```python
from build123d import *

# Parameters (mm, degrees)
SKETCH1_R           = 2
BOSS_EXTRUDE1_DEPTH = 200


with BuildPart() as part:
    # Sketch1 → Boss-Extrude1 (new body)
    with BuildSketch(Plane(origin=(0, 0, 0), x_dir=(1, 0, 0), z_dir=(0, 1, 0))):
        with BuildLine():
            Line((2.824264069, 15.973654403), (5.128427125, 13.669491347))
            ThreePointArc((5.128427125, 13.669491347), (5.99551813, 12.371797952), (6.3, 10.841064222))
            Line((6.3, 10.841064222), (6.3, 9.158935778))
            ThreePointArc((6.3, 9.158935778), (5.99551813, 7.628202048), (5.128427125, 6.330508653))
            Line((5.128427125, 6.330508653), (2.824264069, 4.026345597))
            ThreePointArc((2.824264069, 4.026345597), (2.170389941, 3.896281946), (1.8, 4.450609665))
            Line((1.8, 4.450609665), (1.8, 7))
            ThreePointArc((1.8, 7), (1.653553391, 7.353553391), (1.3, 7.5))
            Line((1.3, 7.5), (0.5, 7.5))
            ThreePointArc((0.5, 7.5), (0.146446609, 7.353553391), (0, 7))
            Line((0, 7), (0, 2))
            ThreePointArc((0, 2), (0.585786438, 0.585786438), (2, 0))
            Line((2, 0), (7, 0))
            ThreePointArc((7, 0), (7.353553391, 0.146446609), (7.5, 0.5))
            Line((7.5, 0.5), (7.5, 1.3))
            ThreePointArc((7.5, 1.3), (7.353553391, 1.653553391), (7, 1.8))
            Line((7, 1.8), (4.450609665, 1.8))
            ThreePointArc((4.450609665, 1.8), (3.896281946, 2.170389941), (4.026345597, 2.824264069))
            Line((4.026345597, 2.824264069), (6.330508653, 5.128427125))
            ThreePointArc((6.330508653, 5.128427125), (7.628202048, 5.99551813), (9.158935778, 6.3))
            Line((9.158935778, 6.3), (10.841064222, 6.3))
            ThreePointArc((10.841064222, 6.3), (12.371797952, 5.99551813), (13.669491347, 5.128427125))
            Line((13.669491347, 5.128427125), (15.973654403, 2.824264069))
            ThreePointArc((15.973654403, 2.824264069), (16.103718054, 2.170389941), (15.549390335, 1.8))
            Line((15.549390335, 1.8), (13, 1.8))
            ThreePointArc((13, 1.8), (12.646446609, 1.653553391), (12.5, 1.3))
            Line((12.5, 1.3), (12.5, 0.5))
            ThreePointArc((12.5, 0.5), (12.646446609, 0.146446609), (13, 0))
            Line((13, 0), (18, 0))
            ThreePointArc((18, 0), (19.414213562, 0.585786438), (20, 2))
            Line((20, 2), (20, 7))
            ThreePointArc((20, 7), (19.853553391, 7.353553391), (19.5, 7.5))
            Line((19.5, 7.5), (18.7, 7.5))
            ThreePointArc((18.7, 7.5), (18.346446609, 7.353553391), (18.2, 7))
            Line((18.2, 7), (18.2, 4.450609665))
            ThreePointArc((18.2, 4.450609665), (17.829610059, 3.896281946), (17.175735931, 4.026345597))
            Line((17.175735931, 4.026345597), (14.871572875, 6.330508653))
            ThreePointArc((14.871572875, 6.330508653), (14.00448187, 7.628202048), (13.7, 9.158935778))
            Line((13.7, 9.158935778), (13.7, 10.841064222))
            ThreePointArc((13.7, 10.841064222), (14.00448187, 12.371797952), (14.871572875, 13.669491347))
            Line((14.871572875, 13.669491347), (17.175735931, 15.973654403))
            ThreePointArc((17.175735931, 15.973654403), (17.829610059, 16.103718054), (18.2, 15.549390335))
            Line((18.2, 15.549390335), (18.2, 13))
            ThreePointArc((18.2, 13), (18.346446609, 12.646446609), (18.7, 12.5))
            Line((18.7, 12.5), (19.5, 12.5))
            ThreePointArc((19.5, 12.5), (19.853553391, 12.646446609), (20, 13))
            Line((20, 13), (20, 18))
            ThreePointArc((20, 18), (19.414213562, 19.414213562), (18, 20))
            Line((18, 20), (13, 20))
            ThreePointArc((13, 20), (12.646446609, 19.853553391), (12.5, 19.5))
            Line((12.5, 19.5), (12.5, 18.7))
            ThreePointArc((12.5, 18.7), (12.646446609, 18.346446609), (13, 18.2))
            Line((13, 18.2), (15.549390335, 18.2))
            ThreePointArc((15.549390335, 18.2), (16.103718054, 17.829610059), (15.973654403, 17.175735931))
            Line((15.973654403, 17.175735931), (13.669491347, 14.871572875))
            ThreePointArc((13.669491347, 14.871572875), (12.371797952, 14.00448187), (10.841064222, 13.7))
            Line((10.841064222, 13.7), (9.158935778, 13.7))
            ThreePointArc((9.158935778, 13.7), (7.628202048, 14.00448187), (6.330508653, 14.871572875))
            Line((6.330508653, 14.871572875), (4.026345597, 17.175735931))
            ThreePointArc((4.026345597, 17.175735931), (3.896281946, 17.829610059), (4.450609665, 18.2))
            Line((4.450609665, 18.2), (7, 18.2))
            ThreePointArc((7, 18.2), (7.353553391, 18.346446609), (7.5, 18.7))
            Line((7.5, 18.7), (7.5, 19.5))
            ThreePointArc((7.5, 19.5), (7.353553391, 19.853553391), (7, 20))
            Line((7, 20), (2, 20))
            ThreePointArc((2, 20), (0.585786438, 19.414213562), (0, 18))
            Line((0, 18), (0, 13))
            ThreePointArc((0, 13), (0.146446609, 12.646446609), (0.5, 12.5))
            Line((0.5, 12.5), (1.3, 12.5))
            ThreePointArc((1.3, 12.5), (1.653553391, 12.646446609), (1.8, 13))
            Line((1.8, 13), (1.8, 15.549390335))
            ThreePointArc((1.8, 15.549390335), (2.170389941, 16.103718054), (2.824264069, 15.973654403))
        make_face()
        with Locations(Location((10, 10, 0), (0, 0, 270))):
            Circle(SKETCH1_R, mode=Mode.SUBTRACT)
    extrude(amount=-BOSS_EXTRUDE1_DEPTH)


solid = part.part
```
Model file for the job. Use its own axes, mm. Round coordinates to 2 decimals unless told otherwise and drop trailing zeros. One line per item, written item: value.
(1) Two-plate mould, pull along X, no slides. Class faces 1 (the flat face through (20, -99, -4)), 2 (the cylindrical face through (12, -99, -10)), 3 (the flat face through (4, -99, 0)), 4 (the flat face through (0, -99, -5)): pulls with the +X half, pulls with the -X half, needs draft (parallel to the pull), parting line crosses it, or undercut.
Values follow:
face 1: pulls with the +X half
face 2: undercut
face 3: needs draft
face 4: pulls with the -X half
(2) Drop flat-ended pins along their axis: P1, Ø1.9, axis at y = -143, z = -10.5, coming from the +X side; P2, Ø0.9, axis at x = 1, y = -79.5, coming from the -Z side; P3, Ø0.8, axis at x = 10, y = -124.5, coming from the -Z side; P4, Ø3, axis at x = 10, z = -10, coming from the -Y side. Give the stop position or say it passes through.
Values follow:
P1: stops at x = 13.75
P2: stops at z = -19.92
P3: stops at z = -13.7
P4: passes through
(3) Wall check: probe 1 along Z at (x, y) = (15.5, -31); probe 2 along Z at (x, y) = (12.75, -182.5); probe 3 along X at (y, z) = (-61.5, -10). Give the ranges that are in metal, low to high.
Values follow:
probe 1: z = -20 to -18.2, -16.7 to -14.3, -5.7 to -3.3, -1.8 to 0
probe 2: z = -19.93 to -18.27, -14.18 to -5.82, -1.73 to -0.07
probe 3: x = 6.3 to 8, 12 to 13.7
